from build123d import *

# Parameters (mm, degrees)
SKETCH1_W           = 20
SKETCH1_H           = 8.1
SKETCH1_W_2         = 18
SKETCH1_H_2         = 6.1
BOSS_EXTRUDE1_DEPTH = 14
CHAMFER1_SIZE       = 0.25


with BuildPart() as part:
    # Sketch1 → Boss-Extrude1 (new body)
    with BuildSketch(Plane.XY):
        Rectangle(SKETCH1_W, SKETCH1_H)
        Rectangle(SKETCH1_W_2, SKETCH1_H_2, mode=Mode.SUBTRACT)
    extrude(amount=BOSS_EXTRUDE1_DEPTH)

    # Chamfer1
    chamfer1_edges = [part.edges().sort_by_distance(p)[0] for p in [
        (9, 0, 0),
        (0, 3.05, 0),
        (-9, 0, 0),
        (0, -3.05, 0),
        (9, 0, 14),
        (0, 3.05, 14),
        (-9, 0, 14),
        (0, -3.05, 14),
    ]]
    chamfer(chamfer1_edges, length=CHAMFER1_SIZE)


solid = part.part
Geometry: final body of the model. Coordinates: model frame, mm. A direction names the side the tool comes from. Coordinates: 2 decimals unless noted, no trailing zeros. Write each loop counter-clockwise with the first axis right and the second up, starting at its lowest first coordinate (ties: lowest second). Pieces come first, ordered by that corner, then holes. Notation, with made-up numbers: (32, -6) - (44, -6) arc R18 ccw to (44, 21) - close; hole circle Ø5 at (75.25, -6). An arc over 180 degrees is marked (long way). Return JSON: item names as keys, results as strings.
Item 1: Reachability of faces 4 (the face through (9, 0, 7)), 5 (the face through (0, 3.6, 0)) from +Z, -Z, +X, -X, +Y, -Y: full face, straight path, thin tool, end or side. Return the list, or none.
Completed:
{"face 4": "+Z, -Z", "face 5": "-Z, +X, -X, +Y, -Y"}
Item 2: Section query B-B (x = 4.5). Output: boundary loops of the cut face in (y, z).
Completed:
{"outline": "(-4.05, 0) - (-3.3, 0) - (-3.05, 0.25) - (-3.05, 13.75) - (-3.3, 14) - (-4.05, 14) - close; (3.05, 0.25) - (3.3, 0) - (4.05, 0) - (4.05, 14) - (3.3, 14) - (3.05, 13.75) - close"}
Item 3: Line query: L1, parallel to Y at x = 2.5, z = 8.75; L2, parallel to X at y = -2.5, z = 5. Output: solid intervals per line, ascending.
Completed:
{"L1": "y = -4.05 to -3.05, 3.05 to 4.05", "L2": "x = -10 to -9, 9 to 10"}
Item 4: Section query A-A (z = 6.5). Output: boundary loops of the cut face in (x, y), and give its area (3 significant figures).
Completed:
{"outline": "(-10, -4.05) - (10, -4.05) - (10, 4.05) - (-10, 4.05) - close; hole (-9, -3.05) - (9, -3.05) - (9, 3.05) - (-9, 3.05) - close", "area": "52.2 mm2"}
Item 5: Section query C-C (y = -2.5). Output: boundary loops of the cut face in (x, z).
Completed:
{"outline": "(-10, 0) - (-9.25, 0) - (-9, 0.25) - (-9, 13.75) - (-9.25, 14) - (-10, 14) - close; (9, 0.25) - (9.25, 0) - (10, 0) - (10, 14) - (9.25, 14) - (9, 13.75) - close"}
Item 6: Pull-direction query (X, two-part tool) for faces 1 (the face through (0, 3.05, 7)), 2 (the face through (-10, 0, 7)), 3 (the face through (0, 4.05, 7)); classes: +X half, -X half, draft (parallel to the pull), parting line (faces both ways), or undercut.
Completed:
{"face 1": "undercut", "face 2": "-X half", "face 3": "draft"}
